from build123d import *

# Parameters (mm, degrees)
F0_W     = 80
F0_H     = 200
F0_W_2   = 39
F0_H_2   = 159
F1_DEPTH = 10
F2_DEPTH = 40


with BuildPart() as f1:
    # F0 (on Top) → F1 (new body)
    with BuildSketch(Plane.XY):
        with Locations((40, 100)):
            Rectangle(F0_W, F0_H)
        with Locations((40, 100)):
            Rectangle(F0_W_2, F0_H_2, mode=Mode.SUBTRACT)
    extrude(amount=F1_DEPTH)

    # F0 (on Top) → F2 (join)
    with BuildSketch(Plane.XY):
        with Locations((40, 100)):
            Rectangle(F0_W_2, F0_H_2)
    extrude(amount=F2_DEPTH)


solid = f1.part
Model file for the job. Use its own axes, mm. A direction names the side the tool comes from. Coordinates: 2 decimals unless noted, no trailing zeros. Order: outer loops, then holes, each group sorted by start corner. A loop starts at its lowest first (then second) coordinate and runs counter-clockwise, first axis right, second up. Notation, with made-up numbers: (2, 15) -> (39, 15) arc R26 ccw to (39, 43) -> close; hole circle Ø6 at (44, 12). An arc over 180 degrees is marked (long way). Return JSON: item names as keys, results as strings. Group by question number.
Item 1: Wall check: line 1 along X through (y, z) = (113, 36); line 2 along Y through (x, z) = (29.5, 16); line 3 along Z through (x, y) = (11, 141). Give the ranges that are in metal, low to high. Write a range as [from, to].
Item 2: Saw through at A-A on y = 98. Write the cut outline in (x, z).
Item 3: Saw through at D-D on y = 15. Write the cut outline in (x, z).
Item 4: Flat gauge pins, fed straight in: P1, Ø9, axis at y = 109, z = 21.5, coming from the -X side; P2, Ø8, axis at x = 58.5, z = 35, coming from the -Y side; P3, Ø9, axis at y = 138.5, z = 26.5, coming from the +X side. Where does each tip first touch, or does it go through?
Item 5: Tool access for faces 1 (the flat face through (40, 20.5, 25)), 2 (the flat face through (59.5, 99, 25)), 3 (the flat face through (20.5, 99, 25)): list every direction of +Z, -Z, +X, -X, +Y, -Y with a clear straight run to the whole face (end or side of a thin tool).
Item 6: Saw through at B-B on x = 51. Write the cut outline in (y, z).
Item 7: Saw through at C-C on z = 14. Write the cut outline in (x, y), then the cut area to 3 significant figures.
Values found:
{
 "1": {"line 1": "x = [20.5, 59.5]", "line 2": "y = [20.5, 179.5]", "line 3": "z = [0, 10]"},
 "2": {"outline": "(0, 0) -> (80, 0) -> (80, 10) -> (59.5, 10) -> (59.5, 40) -> (20.5, 40) -> (20.5, 10) -> (0, 10) -> close"},
 "3": {"outline": "(0, 0) -> (80, 0) -> (80, 10) -> (0, 10) -> close"},
 "4": {"P1": "stops at x = 20.5", "P2": "stops at y = 20.5", "P3": "stops at x = 59.5"},
 "5": {"face 1": "+Z, +X, -X, -Y", "face 2": "+Z, +X, +Y, -Y", "face 3": "+Z, -X, +Y, -Y"},
 "6": {"outline": "(0, 0) -> (200, 0) -> (200, 10) -> (179.5, 10) -> (179.5, 40) -> (20.5, 40) -> (20.5, 10) -> (0, 10) -> close"},
 "7": {"outline": "(20.5, 20.5) -> (59.5, 20.5) -> (59.5, 179.5) -> (20.5, 179.5) -> close", "area": "6,200 mm2"}
}
